Here's how the part is built. I have some questions about the finished solid (model axes, mm). A direction names the side the tool comes from. Give positions to 0.01 mm unless a question says otherwise; leave off trailing zeros. Order: outer loops, then holes, each group sorted by start corner. A loop starts at its lowest first (then second) coordinate and runs counter-clockwise, first axis right, second up.
from build123d import *

# Parameters (mm, degrees)
SKETCH016_W = 3
SKETCH016_H = 10
SKETCH017_W = 1
SKETCH017_H = 9.6
SKETCH025_W = 28
SKETCH025_H = 1
SKETCH024_W = 30
SKETCH024_H = 12


with BuildPart() as part:
    # Sketch016 → AdditiveLoft section 0
    with BuildSketch(Plane.XY.offset(-0.2)):
        Rectangle(SKETCH016_W, SKETCH016_H)
    # Sketch017 → AdditiveLoft section 1
    with BuildSketch(Plane.XY.offset(4.8)):
        Rectangle(SKETCH017_W, SKETCH017_H)
    loft()

    # AdditivePipe001: sweep along a path in Sketch022
    with BuildLine(Plane.XZ) as additivepipe001_path:
        Line((0, -0.2), (0, -29.8))
    # Sketch023 (on Face1 of AdditiveLoft) → AdditivePipe001 (sweep)
    with BuildSketch(Plane(origin=(0, 0, -0.2), x_dir=(1, 0, 0), z_dir=(0, 0, -1))):
        with BuildLine():
            Line((10.5, 27.5), (10.5, -27.5))
            Line((10.5, -27.5), (22.6, -27.5))
            ThreePointArc((-22.6, -27.5), (0, -50.1), (22.6, -27.5))
            Line((-10.5, -27.5), (-22.6, -27.5))
            Line((-10.5, -27.5), (-6.2, -27.5))
            Line((-6.2, -7.2), (-6.2, -27.5))
            Line((-15.2, -7.2), (-6.2, -7.2))
            Line((-15.2, 7.2), (-15.2, -7.2))
            Line((-15.2, 7.2), (-6.2, 7.2))
            Line((-6.2, 7.2), (-6.2, 27.5))
            Line((-6.2, 27.5), (-10.5, 27.5))
            Line((-10.5, 27.5), (-22.6, 27.5))
            ThreePointArc((22.6, 27.5), (0, 50.1), (-22.6, 27.5))
            Line((10.5, 27.5), (22.6, 27.5))
        make_face()
    sweep(path=additivepipe001_path.line)

    # Sketch025 (on Face1 of AdditivePipe001) → SubtractiveLoft005 section 0
    with BuildSketch(Plane.XY.offset(-2.2)):
        Rectangle(SKETCH025_W, SKETCH025_H)
    # Sketch024 (on Face14 of AdditivePipe001) → SubtractiveLoft005 section 1
    with BuildSketch(Plane(origin=(-15.2, 0, -30), x_dir=(1, 0, 0), z_dir=(0, 0, 1))):
        with Locations((13.5, 0)):
            Rectangle(SKETCH024_W, SKETCH024_H)
    loft(mode=Mode.SUBTRACT)

    # SubtractivePipe011: sweep along a path in Sketch043
    with BuildLine(Plane(origin=(0, 0, 0), x_dir=(0, -1, 0), z_dir=(-1, 0, 0))) as subtractivepipe011_path:
        Line((-15, -0.2), (-15, -28.8))
    # Sketch042 → SubtractivePipe011 (sweep, cut)
    with BuildSketch(Plane.XY.offset(-0.2)):
        with BuildLine():
            Line((-5, -7), (-5, -28.6))
            Line((-13.4, -28.6), (-5, -28.6))
            Line((-20.4, -28.6), (-13.4, -28.6))
            ThreePointArc((-20.4, -28.6), (0, -49), (20.4, -28.6))
            Line((20.4, -28.6), (13.4, -28.6))
            Line((9.4, -28.6), (13.4, -28.6))
            Line((9.4, -28.6), (9.4, -7))
            Line((9.4, -7), (-5, -7))
        make_face()
    sweep(path=subtractivepipe011_path.line, mode=Mode.SUBTRACT)

    # SubtractivePipe012: sweep along a path in Sketch043
    with BuildLine(Plane(origin=(0, 0, 0), x_dir=(0, -1, 0), z_dir=(-1, 0, 0))) as subtractivepipe012_path:
        Line((-15, -0.2), (-15, -28.8))
    # Sketch044 → SubtractivePipe012 (sweep, cut)
    with BuildSketch(Plane.XY.offset(-0.2)):
        with BuildLine():
            Line((-5, 28.6), (-5, 7))
            Line((-5, 7), (9.4, 7))
            Line((9.4, 7), (9.4, 28.6))
            Line((9.4, 28.6), (13.4, 28.6))
            Line((13.4, 28.6), (20.4, 28.6))
            ThreePointArc((20.4, 28.6), (0, 49), (-20.4, 28.6))
            Line((-13.4, 28.6), (-20.4, 28.6))
            Line((-5, 28.6), (-13.4, 28.6))
        make_face()
    sweep(path=subtractivepipe012_path.line, mode=Mode.SUBTRACT)


solid = part.part
Q1. Thinking about a two-plate mould opening in Y: for faces 1 (the face through (0, -49, -15)), 2 (the face through (2, -7, -15)), 3 (the face through (0, -28, -29.8)), 4 (the face through (-0.497, 50.095, -15.207)), which applies, released by +Y, released by -Y, zero draft, split by the parting line, or undercut?
Filled sheet:
face 1: undercut
face 2: undercut
face 3: zero draft
face 4: released by +Y
Q2. If we section it at B-B on z = -16: Give the number of separate pieces and of enclosed holes in the cut face, plus the area to 3 significant figures.
Filled sheet:
separate pieces: 2
enclosed holes: 2
area: 557 mm2
Q3. If we section it at A-A on y = 12.5: List the corners of the cut face in (x, z) for me.
Filled sheet:
outline: (-6.2, -29.8) - (10.5, -29.8) - (10.5, -0.2) - (9.4, -0.2) - (9.4, -28.8) - (-5, -28.8) - (-5, -0.2) - (-6.2, -0.2) - close
Q4. For faces 5 (the face through (-5, 18, -15)), 6 (the face through (-11, 7.2, -15)), 7 (the face through (10.5, 6, -15)), which set-ups out of +Z, -Z, +X, -X, +Y, -Y let a thin tool reach every point of the face, with its end or its side?
Filled sheet:
face 5: +Z
face 6: +Z, -Z, -X
face 7: +Z, -Z, +X
Q5. I need wall thicknesses on L1, parallel to Y at x = 4, z = -11; L2, parallel to Y at x = -16, z = -22; L3, parallel to X at y = 12.5, z = -16. Which ranges of each line are inside material? Lowest first, please.
Filled sheet:
L1: y = -49.74 to -48.6, -7 to -2.24, 2.24 to 7, 48.6 to 49.74
L2: y = -43.46 to -41.26, -28.6 to -27.5, 27.5 to 28.6, 41.26 to 43.46
L3: x = -6.2 to -5, 9.4 to 10.5
Q6. I'm going to push flat-ended pins straight in: P1, Ø20.5, axis at x = -3.5, y = 27, coming from the +Z side; P2, Ø4, axis at y = 5.5, z = -15.5, coming from the +X side; P3, Ø0.8, axis at x = -4, y = 0, coming from the -Z side; P4, Ø4.5, axis at y = 0, z = -20.5, coming from the -X side. Where does each tip first touch, or does it pass through?
Filled sheet:
P1: stops at z = -0.2
P2: stops at x = 10.5
P3: stops at z = -2.2
P4: passes through
